```python
from build123d import *

# Parameters (mm, degrees)
F0_W     = 140.8
F0_H     = 66.8
F0_R     = 1.75
F0_R_2   = 3.5
F0_W_2   = 7.5
F0_H_2   = 47.8
F0_H_3   = 7.5
F0_W_3   = 121.8
F1_DEPTH = 10.25
F2_DEPTH = 8.25
F3_R     = 3.5
F4_R     = 3
F5_DEPTH = 3
F6_W     = 36
F6_H     = 6.25
F7_DEPTH = 2


with BuildPart() as f1:
    # F0 (on Top) → F1 (new body)
    with BuildSketch(Plane.XY):
        with Locations((70.4, 33.4)):
            Rectangle(F0_W, F0_H)
        Polygon((2, 57.3), (2, 64.8), (9.5, 64.8), (131.3, 64.8), (138.8, 64.8), (138.8, 57.3), (138.8, 9.5), (138.8, 2), (131.3, 2), (9.5, 2), (2, 2), (2, 9.5), align=None, mode=Mode.SUBTRACT)
        Polygon((131.3, 57.3), (9.5, 57.3), (9.5, 9.5), (131.3, 9.5), (131.3, 13.275), (39.5, 13.275), (39.5, 53.525), (131.3, 53.525), align=None)
        with Locations((21.5, 11.5)):
            Circle(F0_R, mode=Mode.SUBTRACT)
        with Locations((31.5, 11.5)):
            Circle(F0_R, mode=Mode.SUBTRACT)
        with Locations((26, 26)):
            Circle(F0_R_2, mode=Mode.SUBTRACT)
        with Locations((5.75, 33.4)):
            Rectangle(F0_W_2, F0_H_2)
        with Locations((5.75, 61.05)):
            Rectangle(F0_W_2, F0_H_3)
        with Locations((5, 61.8)):
            Circle(F0_R, mode=Mode.SUBTRACT)
        with Locations((70.4, 61.05)):
            Rectangle(F0_W_3, F0_H_3)
        with Locations((135.05, 61.05)):
            Rectangle(F0_W_2, F0_H_3)
        with Locations((135.8, 61.8)):
            Circle(F0_R, mode=Mode.SUBTRACT)
        Polygon((138.8, 57.3), (131.3, 57.3), (131.3, 53.525), (138, 53.525), (138, 13.275), (131.3, 13.275), (131.3, 9.5), (138.8, 9.5), align=None)
        with Locations((135.05, 5.75)):
            Rectangle(F0_W_2, F0_H_3)
        with Locations((135.8, 5)):
            Circle(F0_R, mode=Mode.SUBTRACT)
        with Locations((70.4, 5.75)):
            Rectangle(F0_W_3, F0_H_3)
        with Locations((5.75, 5.75)):
            Rectangle(F0_W_2, F0_H_3)
        with Locations((5, 5)):
            Circle(F0_R, mode=Mode.SUBTRACT)
    extrude(amount=-F1_DEPTH)

    # F0 (on Top) → F2 (cut)
    with BuildSketch(Plane.XY):
        with Locations((70.4, 61.05)):
            Rectangle(F0_W_3, F0_H_3)
        Polygon((131.3, 57.3), (9.5, 57.3), (9.5, 9.5), (131.3, 9.5), (131.3, 13.275), (39.5, 13.275), (39.5, 53.525), (131.3, 53.525), align=None)
        with Locations((21.5, 11.5)):
            Circle(F0_R, mode=Mode.SUBTRACT)
        with Locations((31.5, 11.5)):
            Circle(F0_R, mode=Mode.SUBTRACT)
        with Locations((26, 26)):
            Circle(F0_R_2, mode=Mode.SUBTRACT)
        with Locations((70.4, 5.75)):
            Rectangle(F0_W_3, F0_H_3)
        with Locations((5.75, 33.4)):
            Rectangle(F0_W_2, F0_H_2)
        Polygon((138.8, 57.3), (131.3, 57.3), (131.3, 53.525), (138, 53.525), (138, 13.275), (131.3, 13.275), (131.3, 9.5), (138.8, 9.5), align=None)
    extrude(amount=-F2_DEPTH, mode=Mode.SUBTRACT)

    # F3
    f3_edges = [f1.edges().sort_by_distance(p)[0] for p in [
        (140.8, 66.8, -5.125),
        (0, 66.8, -5.125),
        (0, 0, -5.125),
        (140.8, 0, -5.125),
    ]]
    fillet(f3_edges, radius=F3_R)

    # F4 (on face) → F5 (cut)
    with BuildSketch(Plane(origin=(0, 0, -10.25), x_dir=(1, 0, 0), z_dir=(0, 0, -1))):
        with Locations((5, -5)):
            Circle(F4_R)
        with Locations((135.8, -5)):
            Circle(F4_R)
        with Locations((135.8, -61.8)):
            Circle(F4_R)
        with Locations((5, -61.8)):
            Circle(F4_R)
    extrude(amount=-F5_DEPTH, mode=Mode.SUBTRACT)

    # F6 (on face) → F7 (cut)
    with BuildSketch(Plane(origin=(0, 0, 0), x_dir=(0, -1, 0), z_dir=(-1, 0, 0))):
        with Locations((-39.3, -3.125)):
            Rectangle(F6_W, F6_H)
    extrude(amount=-F7_DEPTH, mode=Mode.SUBTRACT)


solid = f1.part
```
Could you check a few things on this model? Use its own coordinates, in mm. A direction names the side the tool comes from. Round coordinates to 2 decimals unless told otherwise and drop trailing zeros. Write each loop counter-clockwise with the first axis right and the second up, starting at its lowest first coordinate (ties: lowest second). Pieces come first, ordered by that corner, then holes. Notation, with made-up numbers: M 27.25,16 L 46.25,16 A25 ccw 46.25,37 Z; hole C -34,-33 d11. An arc over 180 degrees is marked long. Answer in a Markdown table with one row per item. Add a question column.
Q1. If I drill on line 1 (X direction, y = 5, z = -8.75); line 2 (Y direction, x = 5, z = -8.35); line 3 (Y direction, x = 135.8, z = -8.7) (3 decimals), over which ranges is the centre line in solid material (lowest first)? Write a range as from..to.
Q2. Imagine slicing it at A-A (y = 18). Please give me the cut outline in (x, z).
Q3. If we mould it in two halves opening along X, with no side actions, what happens to faces 1 (the flat face through (0, 26, -7)), 2 (the flat face through (140.8, 33, -5)), 3 (the flat face through (9.5, 6, -4))? For each: +X half, -X half, draft (parallel to the pull), parting line (faces both ways), or undercut.
Q4. On a 3-axis mill with a long thin cutter (end or side, diameter ignored), from which of +Z, -Z, +X, -X, +Y, -Y can I reach the whole of each face in a straight line? I mean faces 4 (the flat face through (69, 66.8, -5)), 5 (the flat face through (131.3, 61, -4)), 6 (the cylindrical face through (132.8, 61.7, -8.8)). Say none if no direction works.
Q5. Imagine slicing it at B-B (x = 93). Please give me the cut outline in (y, z) (3 decimals).
Q6. Imagine slicing it at D-D (x = 135.8). Please give me the cut outline in (y, z) (3 decimals), then the cut area to 3 significant figures.
Q7. Imagine slicing it at C-C (z = -3.75). Please give me the cut outline in (x, y).
Q8. Will this pin go through, and if not, where does the flat tip stop? pin 1 Ø1.8 at (x, y) = (136.5, 62.5) entering from -Z.
Values:
| question | item | result |
|---|---|---|
| 1 | line 1 | 0..2, 8..132.8, 138.8..140.8 |
| 1 | line 2 | 0..2, 8..58.8, 64.8..66.8 |
| 1 | line 3 | 0..2, 8..13.275, 53.525..58.8, 64.8..66.8 |
| 2 | outline | M 0,-10.25 L 39.5,-10.25 L 39.5,-8.25 L 2,-8.25 L 2,0 L 0,0 Z; M 138,-10.25 L 140.8,-10.25 L 140.8,0 L 138.8,0 L 138.8,-8.25 L 138,-8.25 Z |
| 3 | face 1 | -X half |
| 3 | face 2 | +X half |
| 3 | face 3 | undercut |
| 4 | face 4 | +Z, -Z, +X, -X, +Y |
| 4 | face 5 | +Z |
| 4 | face 6 | -Z |
| 5 | outline | M 0,-10.25 L 13.275,-10.25 L 13.275,-8.25 L 2,-8.25 L 2,0 L 0,0 Z; M 53.525,-10.25 L 66.8,-10.25 L 66.8,0 L 64.8,0 L 64.8,-8.25 L 53.525,-8.25 Z |
| 6 | outline | M 0,-10.25 L 2,-10.25 L 2,-7.25 L 3.25,-7.25 L 3.25,0 L 0,0 Z; M 6.75,-7.25 L 8,-7.25 L 8,-10.25 L 13.275,-10.25 L 13.275,-8.25 L 9.5,-8.25 L 9.5,0 L 6.75,0 Z; M 53.525,-10.25 L 58.8,-10.25 L 58.8,-7.25 L 60.05,-7.25 L 60.05,0 L 57.3,0 L 57.3,-8.25 L 53.525,-8.25 Z; M 63.55,-7.25 L 64.8,-7.25 L 64.8,-10.25 L 66.8,-10.25 L 66.8,0 L 63.55,0 Z |
| 6 | area | 123 mm^2 |
| 7 | outline | M 0,3.5 A3.5 ccw 3.5,0 L 137.3,0 A3.5 ccw 140.8,3.5 L 140.8,63.3 A3.5 ccw 137.3,66.8 L 3.5,66.8 A3.5 ccw 0,63.3 L 0,57.3 L 9.5,57.3 L 9.5,64.8 L 131.3,64.8 L 131.3,57.3 L 138.8,57.3 L 138.8,9.5 L 131.3,9.5 L 131.3,2 L 9.5,2 L 9.5,9.5 L 2,9.5 L 2,21.3 L 0,21.3 Z; hole C 5,5 d3.5; hole C 5,61.8 d3.5; hole C 135.8,5 d3.5; hole C 135.8,61.8 d3.5 |
| 8 | pin 1 | z = -7.25 |
